Design review of the part built by this model. Coordinates are the model's own, in mm. Face numbers are marked on the shaded views. A direction names the side the tool comes from. Round coordinates to 2 decimals unless told otherwise and drop trailing zeros. Write each loop counter-clockwise with the first axis right and the second up, starting at its lowest first coordinate (ties: lowest second). Pieces come first, ordered by that corner, then holes.
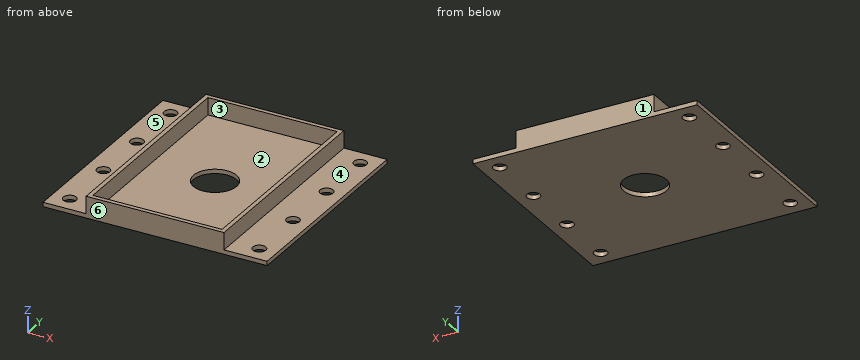
from build123d import *

# Parameters (mm, degrees)
ESQUISSE1_W             = 160
ESQUISSE1_H             = 250
ESQUISSE1_W_2           = 150
ESQUISSE1_H_2           = 240
BOSS_EXTRU_1_DEPTH      = 20
ESQUISSE2_W             = 260
ESQUISSE2_H             = 250
BOSS_EXTRU_2_DEPTH      = 5
ESQUISSE3_R             = 25
ENL_V_MAT_EXTRU_1_DEPTH = 5
ESQUISSE4_R             = 7.5
ENL_V_MAT_EXTRU_2_DEPTH = 10


with BuildPart() as part:
    # Esquisse1 → Boss.-Extru.1 (new body)
    with BuildSketch(Plane.XY):
        with Locations((-80, 125)):
            Rectangle(ESQUISSE1_W, ESQUISSE1_H)
        with Locations((-80, 125)):
            Rectangle(ESQUISSE1_W_2, ESQUISSE1_H_2, mode=Mode.SUBTRACT)
    extrude(amount=BOSS_EXTRU_1_DEPTH)

    # Esquisse2 → Boss.-Extru.2 (add)
    with BuildSketch(Plane(origin=(0, 0, 0), x_dir=(-1, 0, 0), z_dir=(0, 0, -1))):
        with Locations((80, 125)):
            Rectangle(ESQUISSE2_W, ESQUISSE2_H)
    extrude(amount=BOSS_EXTRU_2_DEPTH)

    # Esquisse3 → Enlèv. mat.-Extru.1 (cut)
    with BuildSketch(Plane(origin=(0, 0, -5), x_dir=(-1, 0, 0), z_dir=(0, 0, -1))):
        with Locations((80, 125)):
            Circle(ESQUISSE3_R)
    extrude(amount=-ENL_V_MAT_EXTRU_1_DEPTH, mode=Mode.SUBTRACT)

    # Esquisse4 → Enlèv. mat.-Extru.2 (cut)
    with BuildSketch(Plane.XY):
        with Locations((30, 230)):
            Circle(ESQUISSE4_R)
        with Locations((-190, 230)):
            Circle(ESQUISSE4_R)
        with Locations((-190, 160)):
            Circle(ESQUISSE4_R)
        with Locations((30, 160)):
            Circle(ESQUISSE4_R)
        with Locations((-190, 90)):
            Circle(ESQUISSE4_R)
        with Locations((30, 90)):
            Circle(ESQUISSE4_R)
        with Locations((-190, 20)):
            Circle(ESQUISSE4_R)
        with Locations((30, 20)):
            Circle(ESQUISSE4_R)
    extrude(amount=-ENL_V_MAT_EXTRU_2_DEPTH, mode=Mode.SUBTRACT)


solid = part.part
1) Add section A-A on x = -80. State the section outline as (y, z) points, and give its area (3 significant figures).
2) Add section B-B on y = 160. State the section outline as (x, z) points, and give its area (3 significant figures).
3) For line 1 along Y through (x, z) = (30, -3.4); line 2 along Y through (x, z) = (-106.5, 3.75); line 3 along X through (y, z) = (57.5, 6.25), list the stretches that pass through material, from the lowest coordinate up.
4) Add section D-D on x = 30. State the section outline as (y, z) points.
5) Add section C-C on z = 5.25. State the section outline as (x, y) points.
6) For P1, Ø15, axis at x = -196, y = 166, coming from the +Z side; P2, Ø2, axis at y = 53.5, z = 2, coming from the +X side; P3, Ø2, axis at y = 194, z = 10.5, coming from the -X side, all flat-tipped, find the tip position at first contact; note any pin that passes through.
7) For the marked faces 4, 5 and 6, list the 3-axis set-ups (+Z, -Z, +X, -X, +Y, -Y) from which the entire face can be reached by the end or side of a thin tool; tool diameter is ignored.
8) The part is to be moulded in two halves that separate along X. For the marked faces 1, 2 and 3, say which applies: pulls with the +X half, pulls with the -X half, needs draft (parallel to the pull), parting line crosses it, or undercut.
Computed:
1. outline: (0, -5) - (100, -5) - (100, 0) - (5, 0) - (5, 20) - (0, 20) - close; (150, -5) - (250, -5) - (250, 20) - (245, 20) - (245, 0) - (150, 0) - close
1. area: 1,200 mm2
2. outline: (-210, -5) - (-197.5, -5) - (-197.5, 0) - (-210, 0) - close; (-182.5, -5) - (22.5, -5) - (22.5, 0) - (0, 0) - (0, 20) - (-5, 20) - (-5, 0) - (-155, 0) - (-155, 20) - (-160, 20) - (-160, 0) - (-182.5, 0) - close; (37.5, -5) - (50, -5) - (50, 0) - (37.5, 0) - close
2. area: 1,350 mm2
3. line 1: y = 0 to 12.5, 27.5 to 82.5, 97.5 to 152.5, 167.5 to 222.5, 237.5 to 250
3. line 2: y = 0 to 5, 245 to 250
3. line 3: x = -160 to -155, -5 to 0
4. outline: (0, -5) - (12.5, -5) - (12.5, 0) - (0, 0) - close; (27.5, -5) - (82.5, -5) - (82.5, 0) - (27.5, 0) - close; (97.5, -5) - (152.5, -5) - (152.5, 0) - (97.5, 0) - close; (167.5, -5) - (222.5, -5) - (222.5, 0) - (167.5, 0) - close; (237.5, -5) - (250, -5) - (250, 0) - (237.5, 0) - close
5. outline: (-160, 0) - (0, 0) - (0, 250) - (-160, 250) - close; hole (-155, 5) - (-5, 5) - (-5, 245) - (-155, 245) - close
6. P1: stops at z = 0
6. P2: stops at x = 0
6. P3: stops at x = -160
7. face 4: +Z, +X, +Y, -Y
7. face 5: +Z, -X, +Y, -Y
7. face 6: +Z, -Z, +X, -X, -Y
8. face 1: needs draft
8. face 2: undercut
8. face 3: undercut
